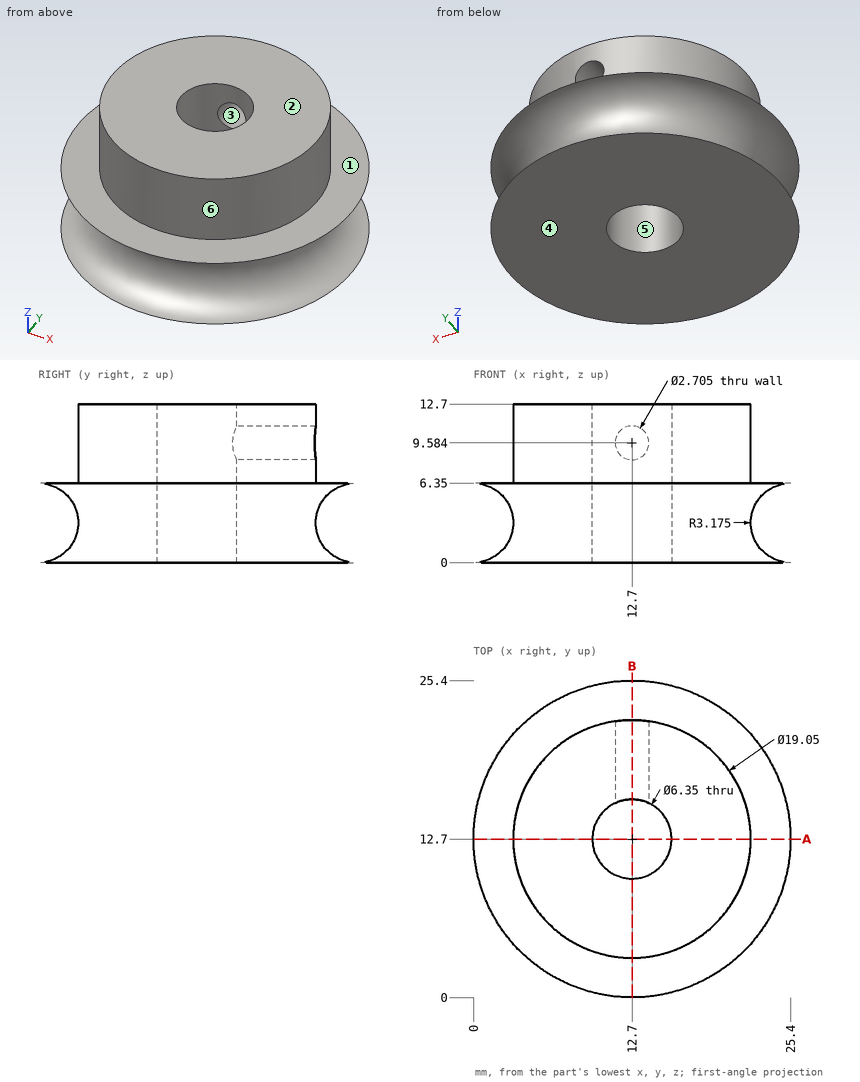
Can you work these out from the drawing? Everything is in mm from the part's minimum corner. A direction names the side the tool comes from. Give positions to 0.01 mm unless a question says otherwise; leave off trailing zeros. Order: outer loops, then holes, each group sorted by start corner. A loop starts at its lowest first (then second) coordinate and runs counter-clockwise, first axis right, second up. Notation, with made-up numbers: M -39,-18.5 L -27,-18.5 A8 cw -27,-7.5 Z; hole C -9,16.25 d10. An arc over 180 degrees is marked long. Use a Markdown table: item, result. Add a question column.
1. I need wall thicknesses on probe 1 along Z at (x, y) = (12.7, 17.5); probe 2 along X at (y, z) = (11, 5.5); probe 3 along X at (y, z) = (10.75, 5.75) (1 decimal). Which ranges of each line are inside material? Lowest first, please. Write a range as from..to.
2. Suppose I cut it at A-A (y = 12.7). List the corners of the cut face in (x, z) for me (3 decimals), and give its area (3 significant figures).
3. Suppose I cut it at B-B (x = 12.7). Give the number of separate pieces and of enclosed holes in the cut face, and give its area (3 significant figures).
4. If we mould it in two halves opening along Y, with no side actions, what happens to the marked faces 4, 5 and 6? For each: +Y half, -Y half, draft (parallel to the pull), parting line (faces both ways), or undercut.
5. For pin 1 Ø2 at (x, z) = (14.5, 7.5) entering from -Y; pin 2 Ø4.5 at (x, z) = (12.7, 9.58) entering from +Y (3 decimals); pin 3 Ø2 at (y, z) = (19, 8) entering from -X; pin 4 Ø10 at (x, y) = (8, 3.5) entering from +Z, each with a flat end and sliding along its axis, tell me the tip position at first contact or that it passes through.
6. On a 3-axis mill with a long thin cutter (end or side, diameter ignored), from which of +Z, -Z, +X, -X, +Y, -Y can I reach the whole of each face in a straight line? I mean the marked faces 1, 2 and 3. Say none if no direction works.
Results list:
| question | item | result |
|---|---|---|
| 1 | probe 1 | z = 0..8.23, 10.94..12.7 |
| 1 | probe 2 | x = 2.3..10.02, 15.38..23.1 |
| 1 | probe 3 | x = 2..10.2, 15.2..23.4 |
| 2 | outline | M 0,0 L 9.525,0 L 9.525,12.7 L 3.175,12.7 L 3.175,6.35 L 0,6.35 A3.175 cw Z; M 15.875,0 L 25.4,0 A3.175 cw 25.4,6.35 L 22.225,6.35 L 22.225,12.7 L 15.875,12.7 Z |
| 2 | area | 170 mm² |
| 3 | separate pieces | 3 |
| 3 | enclosed holes | 0 |
| 3 | area | 153 mm² |
| 4 | face 4 | draft |
| 4 | face 5 | undercut |
| 4 | face 6 | parting line |
| 5 | pin 1 | stops at y = 3.21 |
| 5 | pin 2 | stops at y = 22.225 |
| 5 | pin 3 | stops at x = 4.79 |
| 5 | pin 4 | stops at z = 12.7 |
| 6 | face 1 | +Z |
| 6 | face 2 | +Z, +X, -X, +Y, -Y |
| 6 | face 3 | +Y |
